Autodesk Inventor part; units mm, degrees
ref_plane "YZ Plane" through (0, 0, 0) normal (1, 0, 0) x (0, 1, 0)
ref_plane "XZ Plane" through (0, 0, 0) normal (0, 1, 0) x (-1, 0, 0)
ref_plane "XY Plane" through (0, 0, 0) normal (0, 0, 1) x (1, 0, 0)
sketch "Sketch1" plane through (0, 0, 0) normal (0, 1, 0) x (-1, 0, 0)
  circle A0 centre (0, 0) radius 16
  circle A1 centre (0, -12) radius 2
  circle A2 centre (8.4853, -8.4853) radius 2
  circle A3 centre (12, 0) radius 2
  circle A4 centre (8.4853, 8.4853) radius 2
  circle A5 centre (0, 12) radius 2
  circle A6 centre (-8.4853, 8.4853) radius 2
  circle A7 centre (-12, 0) radius 2
  circle A8 centre (-8.4853, -8.4853) radius 2
  dimension "d0" = 32
  dimension "d1" = 4
  dimension "d2" = 12
  dimension "d5" = 360
extrude "Extrusion1" add sketch "Sketch1" along normal blind 7
properties part number "ArmBearingSpacer2" material "Aluminum 6061"
Build history of the part. All positions in model axes, mm. Round coordinates to 2 decimals unless told otherwise and drop trailing zeros. Order: outer loops, then holes, each group sorted by start corner. A loop starts at its lowest first (then second) coordinate and runs counter-clockwise, first axis right, second up. Notation, with made-up numbers: (25.25, 25.5) -> (33.25, 25.5) arc R17 ccw to (33.25, 37.5) -> close; hole circle Ø3 at (3, 38.25). An arc over 180 degrees is marked (long way). Answer in a Markdown table with one row per item.
1) Pin check, flat tips, straight feed: P1, Ø1, axis at y = 5.5, z = -1.5, coming from the -X side; P2, Ø3, axis at x = 0, z = -12, coming from the +Y side; P3, Ø4, axis at x = 5.5, y = 6, coming from the -Z side; P4, Ø1.5, axis at x = -5.5, y = 6, coming from the +Z side. Stop position of each tip, or through.
Values:
| item | result |
|---|---|
| P1 | x = -15.97 |
| P2 | through |
| P3 | z = -15.61 |
| P4 | z = 15.28 |
2) Band-saw the part on A-A on z = 0. Give the cut face in (x, y), and give its area (3 significant figures).
Values:
| item | result |
|---|---|
| outline | (-16, 0) -> (-14, 0) -> (-14, 7) -> (-16, 7) -> close; (-10, 0) -> (10, 0) -> (10, 7) -> (-10, 7) -> close; (14, 0) -> (16, 0) -> (16, 7) -> (14, 7) -> close |
| area | 168 mm2 |
3) Band-saw the part on B-B on x = 0. Give the cut face in (y, z), and give its area (3 significant figures).
Values:
| item | result |
|---|---|
| outline | (0, -16) -> (7, -16) -> (7, -14) -> (0, -14) -> close; (0, -10) -> (7, -10) -> (7, 10) -> (0, 10) -> close; (0, 14) -> (7, 14) -> (7, 16) -> (0, 16) -> close |
| area | 168 mm2 |
4) Mould opens along X. For faces 1 (the cylindrical face through (6.58, 3.45, 7.88)), 2 (the cylindrical face through (-10.4, 3.5, 1.2)), 3 (the flat face through (0, 7, 0)), 4 (the cylindrical face through (3.47, 3.45, 15.62)) say: released by +X, released by -X, zero draft, split by the parting line, or undercut.
Values:
| item | result |
|---|---|
| face 1 | undercut |
| face 2 | undercut |
| face 3 | zero draft |
| face 4 | split by the parting line |
5) Band-saw the part on D-D on x = 12. Give the cut face in (y, z), and give its area (3 significant figures).
Values:
| item | result |
|---|---|
| outline | (0, -10.58) -> (7, -10.58) -> (7, -2) -> (0, -2) -> close; (0, 2) -> (7, 2) -> (7, 10.58) -> (0, 10.58) -> close |
| area | 120 mm2 |
6) Band-saw the part on C-C on z = 12. Give the cut face in (x, y), and give its area (3 significant figures).
Values:
| item | result |
|---|---|
| outline | (-10.58, 0) -> (-2, 0) -> (-2, 7) -> (-10.58, 7) -> close; (2, 0) -> (10.58, 0) -> (10.58, 7) -> (2, 7) -> close |
| area | 120 mm2 |
7) Wall check: L1, parallel to Z at x = 0, y = 3.75; L2, parallel to X at y = 5.25, z = 9; L3, parallel to X at y = 2.25, z = 8. Give the ranges that are in metal, low to high.
Values:
| item | result |
|---|---|
| L1 | -16 to -14, -10 to 10, 14 to 16 |
| L2 | -13.23 to -10.42, -6.55 to 6.55, 10.42 to 13.23 |
| L3 | -13.86 to -10.43, -6.55 to 6.55, 10.43 to 13.86 |
